Check sheet for the drawn part. Datum: minimum x, y, z corner. Units: mm. A direction names the side the tool comes from. Give positions to 0.01 mm unless a question says otherwise; leave off trailing zeros. Loops run counter-clockwise (first coordinate to the right, second up) from the corner with the lowest first, then second, coordinate; pieces in that order, holes last.
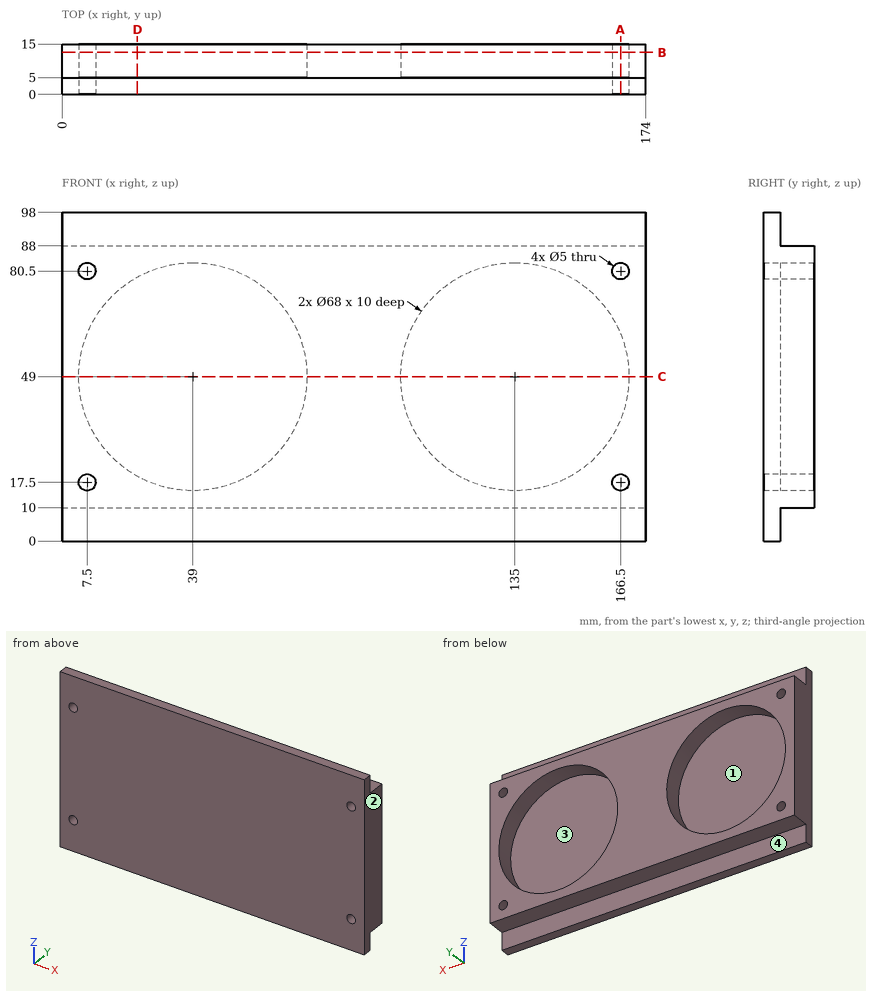
(1) Release check for a two-part mould opening along Z. For the marked faces 3 and 4 record: pulls with the +Z half, pulls with the -Z half, needs draft (parallel to the pull), parting line crosses it, or undercut.
(2) Gauge pin test, flat ends, axial feed: pin 1 Ø3 at (x, y) = (66.5, 7.5) entering from +Z; pin 2 Ø3 at (x, z) = (119.5, 6) entering from +Y. Record the tip position at first contact, or that the pin passes through.
(3) Section check C-C on z = 49. Record the boundary of the cut face in (x, y).
(4) Access from +Z, -Z, +X, -X, +Y, -Y to the whole of each face (thin tool, end or side, straight path). Record for the marked faces 1 and 2.
(5) Section check A-A on x = 166.5. Record the boundary of the cut face in (y, z), plus the area to 3 significant figures.
(6) Material ranges on line 1 (X direction, y = 9.5, z = 49); line 2 (Z direction, x = 166.5, y = 12); line 3 (X direction, y = 13.75, z = 34.5), recorded low to high.
(7) Section check D-D on x = 22.5. Record the boundary of the cut face in (y, z).
(8) Section check B-B on y = 12.5. Record the boundary of the cut face in (x, z).
Computed values:
1. face 3: undercut
1. face 4: needs draft
2. pin 1: stops at z = 88
2. pin 2: stops at y = 5
3. outline: (0, 0) - (174, 0) - (174, 15) - (169, 15) - (169, 5) - (101, 5) - (101, 15) - (73, 15) - (73, 5) - (5, 5) - (5, 15) - (0, 15) - close
4. face 1: +Y
4. face 2: +Z, -Z, +X, +Y, -Y
5. outline: (0, 0) - (5, 0) - (5, 10) - (15, 10) - (15, 15) - (0, 15) - close; (0, 20) - (15, 20) - (15, 36.2) - (5, 36.2) - (5, 61.8) - (15, 61.8) - (15, 78) - (0, 78) - close; (0, 83) - (15, 83) - (15, 88) - (5, 88) - (5, 98) - (0, 98) - close
5. area: 864 mm2
6. line 1: x = 0 to 5, 73 to 101, 169 to 174
6. line 2: z = 10 to 15, 20 to 36.2, 61.8 to 78, 83 to 88
6. line 3: x = 0 to 8.25, 69.75 to 104.25, 165.75 to 174
7. outline: (0, 0) - (5, 0) - (5, 10) - (15, 10) - (15, 19.27) - (5, 19.27) - (5, 78.73) - (15, 78.73) - (15, 88) - (5, 88) - (5, 98) - (0, 98) - close
8. outline: (0, 10) - (174, 10) - (174, 88) - (0, 88) - close; hole circle Ø5 at (7.5, 17.5); hole circle Ø68 at (39, 49); hole circle Ø5 at (7.5, 80.5); hole circle Ø68 at (135, 49); hole circle Ø5 at (166.5, 17.5); hole circle Ø5 at (166.5, 80.5)
